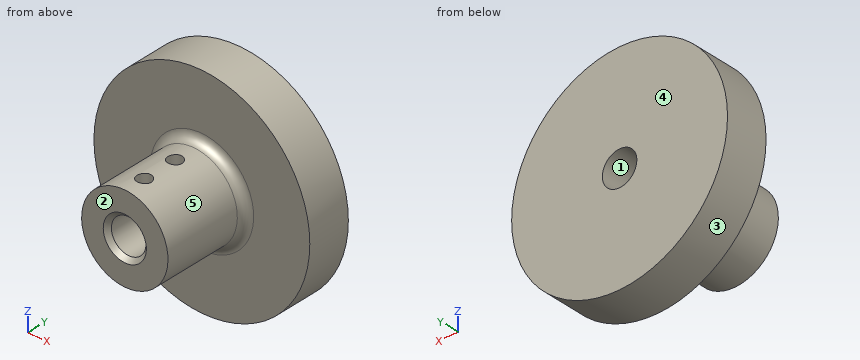
```python
from build123d import *

# Parameters (mm, degrees)
SKETCH1_R                  = 25
BOSS_EXTRUDE1_DEPTH        = 30
CUT_EXTRUDE1_REACH         = 48.368
SKETCH2_R                  = 4
SKETCH3_OUTSIDE_W          = 67.362
SKETCH3_OUTSIDE_H          = 67.362
SKETCH3_OUTSIDE_R          = 10
CUT_EXTRUDE2_DEPTH         = 20
SKETCH4_W                  = 1.65
SKETCH4_H                  = 10
M4_TAPPED_HOLE1_AT_2_COUNT = 2
M4_TAPPED_HOLE1_AT_2_PITCH = 8
CHAMFER1_SIZE              = 1
FILLET1_R                  = 2


with BuildPart() as part:
    # Sketch1 → Boss-Extrude1 (new body)
    with BuildSketch(Plane(origin=(0, 0, 0), x_dir=(1, 0, 0), z_dir=(0, 1, 0))):
        with Locations(Location((0, 0, 0), (0, 0, 270))):
            Circle(SKETCH1_R)
    extrude(amount=BOSS_EXTRUDE1_DEPTH)

    # Sketch2 → Cut-Extrude1 (cut, up to next)
    with BuildSketch(Plane.XZ, mode=Mode.PRIVATE) as cut_extrude1_sk1:
        with Locations(Location((0, 0, 0), (0, 0, 270))):
            Circle(SKETCH2_R)
    cut_extrude1_tool1 = extrude(cut_extrude1_sk1.sketch, amount=-CUT_EXTRUDE1_REACH, mode=Mode.PRIVATE) & part.part
    add(cut_extrude1_tool1.solids().sort_by_distance((0, 0, 0))[0], mode=Mode.SUBTRACT)

    # Sketch3 outside → Cut-Extrude2 (cut)
    with BuildSketch(Plane.XZ):
        Rectangle(SKETCH3_OUTSIDE_W, SKETCH3_OUTSIDE_H)
        with Locations(Location((0, 0, 0), (0, 0, 270))):
            Circle(SKETCH3_OUTSIDE_R, mode=Mode.SUBTRACT)
    extrude(amount=-CUT_EXTRUDE2_DEPTH, mode=Mode.SUBTRACT)

    # Sketch4 → M4 Tapped Hole1 (revolve, cut)
    with BuildSketch(Plane(origin=(0, 5, 0), x_dir=(0, 1, 0), z_dir=(1, 0, 0))):
        with Locations((0.825, 5)):
            Rectangle(SKETCH4_W, SKETCH4_H)
    m4_tapped_hole1 = revolve(axis=Axis((0, 5, -6.35), (0, 0, 1)), mode=Mode.SUBTRACT)

    # M4 Tapped Hole1 at 2: M4 Tapped Hole1 ×2
    with Locations(*[(0, i * M4_TAPPED_HOLE1_AT_2_PITCH, 0) for i in range(1, M4_TAPPED_HOLE1_AT_2_COUNT)]):
        add(m4_tapped_hole1, mode=Mode.SUBTRACT)

    # Chamfer1
    chamfer1_edges = [part.edges().sort_by_distance(p)[0] for p in [
        (0, 0, 4),
    ]]
    chamfer(chamfer1_edges, length=CHAMFER1_SIZE)

    # Fillet1
    fillet1_edges = [part.edges().sort_by_distance(p)[0] for p in [
        (0, 20, 10),
    ]]
    fillet(fillet1_edges, radius=FILLET1_R)


solid = part.part
```
Verification items for the finished model (mm, model axes). Face numbers are marked on the shaded views. A direction names the side the tool comes from. Give positions to 0.01 mm unless a question says otherwise; leave off trailing zeros. Order: outer loops, then holes, each group sorted by start corner. A loop starts at its lowest first (then second) coordinate and runs counter-clockwise, first axis right, second up. Notation, with made-up numbers: M 29.5,50 L 40.5,50 A25 ccw 40.5,74 Z; hole C 57,60.25 d4. An arc over 180 degrees is marked long. Answer in a Markdown table with one row per item. Add a question column.
Item 1: Section check B-B, the plane z = 0. Enter the section's corners in (x, y), and give its area (3 significant figures).
Item 2: Section check D-D, the plane x = -20. Enter the section's corners in (y, z).
Item 3: Gauge pin test, flat ends, axial feed: pin 1 (4 mm diameter, centred on x = 0, y = 13, fed in from +Z); pin 2 (6 mm diameter, centred on y = 26, z = -2, fed in from -X); pin 3 (8 mm diameter, centred on y = 11, z = 10, fed in from +X); pin 4 (7 mm diameter, centred on x = 0, z = 0, fed in from -Y). Record the tip position at first contact, or that the pin passes through.
Item 4: Tool access check on the marked faces 4 and 5. Record the directions out of +Z, -Z, +X, -X, +Y, -Y that give a thin tool (end or side, any length) a straight path to the whole face; none if there is none.
Item 5: Mould release check, pull along Z, two halves, no side actions. Record for the marked faces 1, 2 and 3: released by +Z, released by -Z, zero draft, split by the parting line, or undercut.
Item 6: Scan lines: probe 1 along Z at (x, y) = (0, 21); probe 2 along Z at (x, y) = (0, 11). Record each from-to range of solid material in increasing order. Write a range as from..to.
Item 7: Section check C-C, the plane y = 8.5. Enter the section's corners in (x, z).
Item 8: Section check A-A, the plane x = 0. Enter the section's corners in (y, z).
Filled sheet:
| question | item | result |
|---|---|---|
| 1 | outline | M -25,20 L -12,20 A2 cw -10,18 L -10,0 L -5,0 L -4,1 L -4,30 L -25,30 Z; M 4,1 L 5,0 L 10,0 L 10,18 A2 cw 12,20 L 25,20 L 25,30 L 4,30 Z |
| 1 | area | 661 mm^2 |
| 2 | outline | M 20,-15 L 30,-15 L 30,15 L 20,15 Z |
| 3 | pin 1 | stops at z = 10 |
| 3 | pin 2 | stops at x = -25 |
| 3 | pin 3 | stops at x = 8 |
| 3 | pin 4 | passes through |
| 4 | face 4 | +Z, -Z, +X, -X, +Y |
| 4 | face 5 | -Y |
| 5 | face 1 | undercut |
| 5 | face 2 | zero draft |
| 5 | face 3 | split by the parting line |
| 6 | probe 1 | z = -25..-4, 4..25 |
| 6 | probe 2 | z = -10..-4, 4..10 |
| 7 | outline | C 0,0 d20; hole C 0,0 d8 |
| 8 | outline | M 0,-10 L 18,-10 A2 cw 20,-12 L 20,-25 L 30,-25 L 30,-4 L 1,-4 L 0,-5 Z; M 0,5 L 1,4 L 3.35,4 L 3.35,10 L 0,10 Z; M 6.65,4 L 11.35,4 L 11.35,10 L 6.65,10 Z; M 14.65,4 L 30,4 L 30,25 L 20,25 L 20,12 A2 cw 18,10 L 14.65,10 Z |
